from build123d import *

# Parameters (mm, degrees)
SKETCH1_W           = 15.24
SKETCH1_H           = 25.4
BOSS_EXTRUDE1_DEPTH = 1
FILLET1_R           = 2
SKETCH2_R           = 1.25
SKETCH2_R_2         = 0.508
CUT_EXTRUDE1_DEPTH  = 1
SKETCH3_R           = 5
BOSS_EXTRUDE2_DEPTH = 5
FILLET2_R           = 0.5


with BuildPart() as part:
    # Sketch1 → Boss-Extrude1 (new body)
    with BuildSketch(Plane(origin=(0, 0, 0), x_dir=(1, 0, 0), z_dir=(0, 1, 0))):
        with Locations((-7.62, 12.7)):
            Rectangle(SKETCH1_W, SKETCH1_H)
    extrude(amount=BOSS_EXTRUDE1_DEPTH)

    # Fillet1
    fillet1_edges = [part.edges().sort_by_distance(p)[0] for p in [
        (0, 0.5, 0),
        (-15.24, 0.5, 0),
        (-15.24, 0.5, -25.4),
        (0, 0.5, -25.4),
    ]]
    fillet(fillet1_edges, radius=FILLET1_R)

    # Sketch2 → Cut-Extrude1 (cut)
    with BuildSketch(Plane(origin=(0, 1, 0), x_dir=(1, 0, 0), z_dir=(0, 1, 0))):
        with Locations(Location((-2.5, 22.9, 0), (0, 0, 270))):
            Circle(SKETCH2_R)
        with Locations(Location((-12.74, 22.9, 0), (0, 0, 270))):
            Circle(SKETCH2_R)
        with Locations(Location((-12.62, 2, 0), (0, 0, 270))):
            Circle(SKETCH2_R_2)
        with Locations(Location((-10.12, 2, 0), (0, 0, 270))):
            Circle(SKETCH2_R_2)
        with Locations(Location((-7.62, 2, 0), (0, 0, 270))):
            Circle(SKETCH2_R_2)
        with Locations(Location((-5.12, 2, 0), (0, 0, 270))):
            Circle(SKETCH2_R_2)
        with Locations(Location((-2.62, 2, 0), (0, 0, 270))):
            Circle(SKETCH2_R_2)
    extrude(amount=-CUT_EXTRUDE1_DEPTH, mode=Mode.SUBTRACT)

    # Sketch3 → Boss-Extrude2 (add)
    with BuildSketch(Plane(origin=(0, 1, 0), x_dir=(1, 0, 0), z_dir=(0, 1, 0))):
        with Locations(Location((-7.62, 17.9, 0), (0, 0, 270))):
            Circle(SKETCH3_R)
    extrude(amount=BOSS_EXTRUDE2_DEPTH)

    # Fillet2
    fillet2_edges = [part.edges().sort_by_distance(p)[0] for p in [
        (-7.62, 6, -22.9),
    ]]
    fillet(fillet2_edges, radius=FILLET2_R)


solid = part.part
The listing builds one solid part. Answer for the finished solid, in the listing's coordinates (mm). A direction names the side the tool comes from. Coordinates: 2 decimals unless noted, no trailing zeros. Loops run counter-clockwise (first coordinate to the right, second up) from the corner with the lowest first, then second, coordinate; pieces in that order, holes last.
1) Find section A-A on z = -17.9. Write down the section's boundary in (x, y), then the cut area to 3 significant figures.
2) A tool of negligible diameter and unlimited length cuts with its end or side. For faces 1 (the face through (-14.67, 0.51, -0.6)), 2 (the face through (-7.4, 3.218, -22.895)), from which of +Z, -Z, +X, -X, +Y, -Y can it reach the whole face along a straight path? Write none if from no direction.
3) Find the intervals of material crossed by L1, parallel to X at y = 0.4, z = -22.9; L2, parallel to Z at x = -7.5, y = 4; L3, parallel to Y at x = -0.75, z = -14.5, in increasing order.
4) Flat-ended cylindrical pins translate along their axes: pin 1 Ø1.2 at (x, z) = (-10.12, -2) entering from +Y; pin 2 Ø2 at (x, y) = (-3, 3.5) entering from +Z; pin 3 Ø1 at (x, y) = (-5.5, 4) entering from -Z. Find the tip coordinate at first contact, or state that the pin passes through.
5) Determine the mould class of faces 3 (the face through (-7.7, 0.5, 0)), 4 (the face through (-7.19, 0.51, -1.73)), 5 (the face through (-7.7, 0.5, -25.4)), 6 (the face through (-12.69, 0.51, -24.15)) for opening direction Z: pulls with the +Z half, pulls with the -Z half, needs draft (parallel to the pull), parting line crosses it, or undercut.
6) Find section B-B on y = 3.7. Write down the section's boundary in (x, z), then the cut area to 3 significant figures.
7) Find section C-C on x = -0.75. Write down the section's boundary in (y, z).
8) Find section D-D on z = -9. Write down the section's boundary in (x, y), then the cut area to 3 significant figures.
Values:
1. outline: (-15.24, 0) - (0, 0) - (0, 1) - (-2.62, 1) - (-2.62, 5.5) arc R0.5 ccw to (-3.12, 6) - (-12.12, 6) arc R0.5 ccw to (-12.62, 5.5) - (-12.62, 1) - (-15.24, 1) - close
1. area: 65.1 mm2
2. face 1: +Z, -X, +Y, -Y
2. face 2: +Y
3. L1: x = -15.24 to -13.99, -11.49 to -3.75, -1.25 to 0
3. L2: z = -22.9 to -12.9
3. L3: y = 0 to 1
4. pin 1: stops at y = 1
4. pin 2: stops at z = -14.45
4. pin 3: stops at z = -22.63
5. face 3: pulls with the +Z half
5. face 4: undercut
5. face 5: pulls with the -Z half
5. face 6: undercut
6. outline: circle Ø10 at (-7.62, -17.9)
6. area: 78.5 mm2
7. outline: (0, -24.96) - (1, -24.96) - (1, -0.44) - (0, -0.44) - close
8. outline: (-15.24, 0) - (0, 0) - (0, 1) - (-15.24, 1) - close
8. area: 15.2 mm2
